The drawing under review shows one solid part. Ordinate dimensions are in mm from its lowest x, y, z. A direction names the side the tool comes from. Round coordinates to 2 decimals unless told otherwise and drop trailing zeros. Write each loop counter-clockwise with the first axis right and the second up, starting at its lowest first coordinate (ties: lowest second). Pieces come first, ordered by that corner, then holes. Notation, with made-up numbers: (27, -31.5) -> (56, -31.5) arc R14 ccw to (56, -16.5) -> close; hole circle Ø2 at (-2, -5.75). An arc over 180 degrees is marked (long way). Answer in a Markdown table with one row per item.
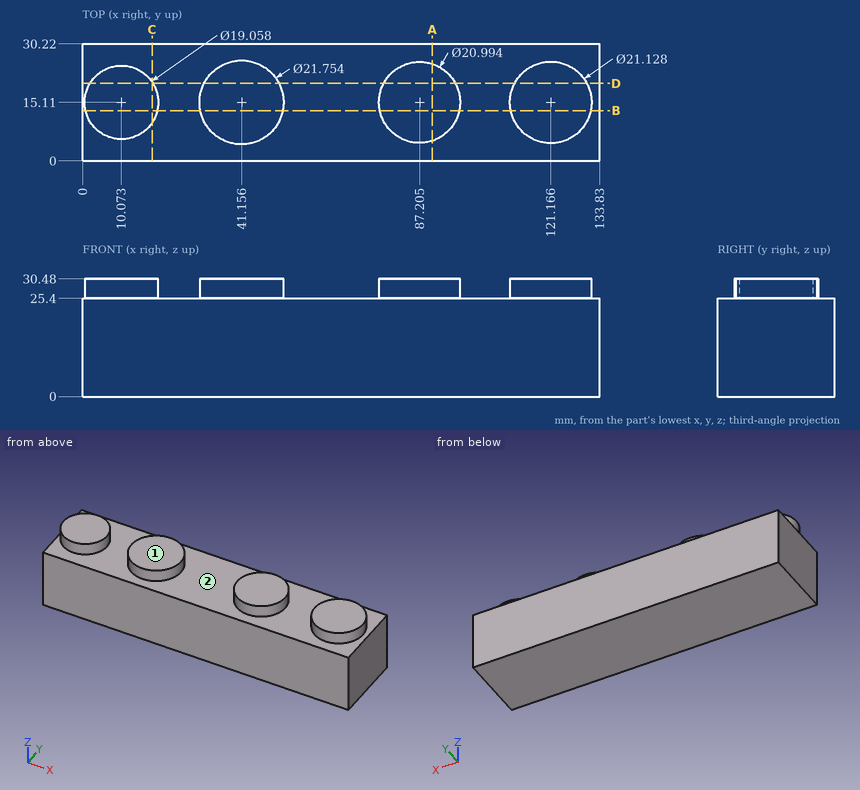
1) For the marked faces 1 and 2, list the 3-axis set-ups (+Z, -Z, +X, -X, +Y, -Y) from which the entire face can be reached by the end or side of a thin tool; tool diameter is ignored.
Solved:
| item | result |
|---|---|
| face 1 | +Z, +X, -X, +Y, -Y |
| face 2 | +Z |
2) Consider section A-A on x = 90.5. State the section outline as (y, z) points.
Solved:
| item | result |
|---|---|
| outline | (0, 0) -> (30.22, 0) -> (30.22, 25.4) -> (25.08, 25.4) -> (25.08, 30.48) -> (5.14, 30.48) -> (5.14, 25.4) -> (0, 25.4) -> close |
3) Consider section B-B on y = 13. State the section outline as (x, z) points (1 decimal), then the cut area to 3 significant figures.
Solved:
| item | result |
|---|---|
| outline | (0, 0) -> (133.8, 0) -> (133.8, 25.4) -> (131.5, 25.4) -> (131.5, 30.5) -> (110.8, 30.5) -> (110.8, 25.4) -> (97.5, 25.4) -> (97.5, 30.5) -> (76.9, 30.5) -> (76.9, 25.4) -> (51.8, 25.4) -> (51.8, 30.5) -> (30.5, 30.5) -> (30.5, 25.4) -> (19.4, 25.4) -> (19.4, 30.5) -> (0.8, 30.5) -> (0.8, 25.4) -> (0, 25.4) -> close |
| area | 3,810 mm² |
4) For line 1 (X direction, y = 15, z = 29) (1 decimal); line 2 (X direction, y = 17, z = 29.5) (1 decimal); line 3 (Z direction, x = 42, y = 27.5), list the stretches that pass through material, from the lowest coordinate up. Write a range as [from, to].
Solved:
| item | result |
|---|---|
| line 1 | [0.5, 19.6], [30.3, 52], [76.7, 97.7], [110.6, 131.7] |
| line 2 | [0.7, 19.4], [30.4, 51.9], [76.9, 97.5], [110.8, 131.6] |
| line 3 | [0, 25.4] |
5) Consider section D-D on y = 20. State the section outline as (x, z) points (1 decimal), then the cut area to 3 significant figures.
Solved:
| item | result |
|---|---|
| outline | (0, 0) -> (133.8, 0) -> (133.8, 25.4) -> (130.5, 25.4) -> (130.5, 30.5) -> (111.8, 30.5) -> (111.8, 25.4) -> (96.5, 25.4) -> (96.5, 30.5) -> (77.9, 30.5) -> (77.9, 25.4) -> (50.9, 25.4) -> (50.9, 30.5) -> (31.4, 30.5) -> (31.4, 25.4) -> (18.3, 25.4) -> (18.3, 30.5) -> (1.9, 30.5) -> (1.9, 25.4) -> (0, 25.4) -> close |
| area | 3,770 mm² |
6) Consider section C-C on x = 18. State the section outline as (y, z) points.
Solved:
| item | result |
|---|---|
| outline | (0, 0) -> (30.22, 0) -> (30.22, 25.4) -> (20.4, 25.4) -> (20.4, 30.48) -> (9.82, 30.48) -> (9.82, 25.4) -> (0, 25.4) -> close |
